```python
from build123d import *

# Parameters (mm, degrees)
EXTRUDE_1_DEPTH          = 15
CUT_EXTRUDE_1_DEPTH      = 15
CUT_EXTRUDE_1_DEPTH_BACK = 15
SKETCH_2_R               = 2.25
CUT_EXTRUDE_2_DEPTH      = 1.5
CUT_EXTRUDE_3_DEPTH      = 1.5
FILLET_1_R               = 0.5
FILLET_2_R               = 1


with BuildPart() as part:
    # Эскиз1 → Вытянуть1 (new body)
    with BuildSketch(Plane.XY):
        with BuildLine():
            Line((-25.229060352, 2.359412), (-25.229060352, 8.559412))
            ThreePointArc((-25.229060352, 8.559412), (-24.666370719, 9.730500928), (-23.400461317, 10.022977057))
            Line((-23.400461317, 10.022977057), (-5.12659913, 5.920136906))
            ThreePointArc((-5.12659913, 5.920136906), (-4.279542261, 5.877403833), (-3.466943303, 6.120332607))
            Line((-3.466943303, 6.120332607), (-1.866464924, 6.915175876))
            Line((-1.866464924, 6.915175876), (-1.510627877, 6.19867047))
            Line((-1.510627877, 6.19867047), (-3.111106257, 5.403827201))
            ThreePointArc((-3.111106257, 5.403827201), (-4.183736881, 5.083161219), (-5.301851949, 5.139568876))
            Line((-5.301851949, 5.139568876), (-23.575714136, 9.242409026))
            ThreePointArc((-23.575714136, 9.242409026), (-24.166471856, 9.105920166), (-24.429060352, 8.559412))
            Line((-24.429060352, 8.559412), (-24.429060352, 2.359412))
            ThreePointArc((-24.429060352, 2.359412), (-25.102714755, 0.733066403), (-26.729060352, 0.059412))
            Line((-26.729060352, 0.059412), (-33.229060352, 0.059412))
            Line((-33.229060352, 0.059412), (-33.229060352, 0.859412))
            Line((-33.229060352, 0.859412), (-26.729060352, 0.859412))
            ThreePointArc((-26.729060352, 0.859412), (-25.66840018, 1.298751828), (-25.229060352, 2.359412))
        make_face()
    extrude(amount=EXTRUDE_1_DEPTH)

    # Эскиз2 → Вырез-Вытянуть1 (cut, two sides: drawn at the far end of the back side and taken through both)
    with BuildSketch(Plane(origin=(0, 0.859412, 0), x_dir=(1, 0, 0), z_dir=(0, 1, 0)).offset(-CUT_EXTRUDE_1_DEPTH_BACK)):
        with Locations(Location((-29.629060352, -7.5, 0), (0, 0, 90))):
            Circle(SKETCH_2_R)
        Polygon((-13.229060352, -0.5), (-13.229060352, -2), (-0.791842207, -2), (-0.791842207, 0), (-26.729060352, 0), (-26.729060352, -0.5), align=None)
        Polygon((-26.729060352, -15), (-0.791842207, -15), (-0.791842207, -13), (-13.229060352, -13), (-13.229060352, -14.5), (-26.729060352, -14.5), align=None)
    extrude(amount=CUT_EXTRUDE_1_DEPTH + CUT_EXTRUDE_1_DEPTH_BACK, mode=Mode.SUBTRACT)

    # Эскиз3 → Вырез-Вытянуть2 (cut)
    with BuildSketch(Plane.XY.offset(14.5)):
        Polygon((-13.229060352, 7.739298224), (-13.229060352, 6.919382502), (-13.40431317, 6.958730194), align=None)
    extrude(amount=-CUT_EXTRUDE_2_DEPTH, mode=Mode.SUBTRACT)

    # Эскиз4 → Вырез-Вытянуть3 (cut)
    with BuildSketch(Plane(origin=(0, 0, 0.5), x_dir=(-1, 0, 0), z_dir=(0, 0, -1))):
        Polygon((13.229060352, 7.739298224), (13.229060352, 6.919382502), (13.40431317, 6.958730194), align=None)
    extrude(amount=-CUT_EXTRUDE_3_DEPTH, mode=Mode.SUBTRACT)

    # Скругление1
    # the kernel refuses this fillet: 0.5 mm, written as the material it adds along each edge
    with BuildSketch(Plane(origin=(-26.729060352, 2.109412, 14.5), x_dir=(0, 0, 1), z_dir=(0, -1, 0))) as fillet_1_piece_1_section:
        with BuildLine():
            CenterArc((FILLET_1_R, -FILLET_1_R), FILLET_1_R, 90, 90)
            Line((0, -FILLET_1_R), (0, 0))
            Line((0, 0), (FILLET_1_R, 0))
        make_face()
    fillet_1_piece_1 = extrude(amount=3.3, mode=Mode.PRIVATE)
    fillet_1_piece_1 = fillet_1_piece_1 - Plane(origin=(-26.729060352, 2.359412, 14.543282734), x_dir=(0, -1, 0), z_dir=(0, 0, -1)) * Cylinder(1.5, 9, mode=Mode.PRIVATE)
    fillet_1_piece_1 = fillet_1_piece_1 & Plane(origin=(-26.729060352, 2.359412, 14.543282734), x_dir=(1, 0, 0), z_dir=(0, 0, -1)) * Cylinder(2.3, 9, mode=Mode.PRIVATE)
    add(fillet_1_piece_1)
    with BuildSketch(Plane(origin=(-26.729060352, 2.109412, 0.5), x_dir=(0, 0, -1), z_dir=(0, -1, 0))) as fillet_1_piece_2_section:
        with BuildLine():
            CenterArc((FILLET_1_R, FILLET_1_R), FILLET_1_R, 180, 90)
            Line((0, FILLET_1_R), (0, 0))
            Line((0, 0), (FILLET_1_R, 0))
        make_face()
    fillet_1_piece_2 = extrude(amount=3.3, mode=Mode.PRIVATE)
    fillet_1_piece_2 = fillet_1_piece_2 - Plane(origin=(-26.729060352, 2.359412, 0.456717266), x_dir=(0, -1, 0), z_dir=(0, 0, -1)) * Cylinder(1.5, 9, mode=Mode.PRIVATE)
    fillet_1_piece_2 = fillet_1_piece_2 & Plane(origin=(-26.729060352, 2.359412, 0.456717266), x_dir=(1, 0, 0), z_dir=(0, 0, -1)) * Cylinder(2.3, 9, mode=Mode.PRIVATE)
    add(fillet_1_piece_2)

    # Скругление2
    fillet_2_edges = [part.edges().sort_by_distance(p)[0] for p in [
        (-1.6885464, 6.556923173, 13),
        (-13.316686761, 7.349014209, 13),
        (-13.316686761, 7.349014209, 2),
        (-1.6885464, 6.556923173, 2),
    ]]
    fillet(fillet_2_edges, radius=FILLET_2_R)


solid = part.part
```
Design review of the part built by this model. Coordinates are the model's own, in mm. A direction names the side the tool comes from. Give positions to 0.01 mm unless a question says otherwise; leave off trailing zeros. Loops run counter-clockwise (first coordinate to the right, second up) from the corner with the lowest first, then second, coordinate; pieces in that order, holes last. Notation, with made-up numbers: (17.5, 44.5) -> (45.5, 44.5) arc R5 ccw to (45.5, 52.5) -> close; hole circle Ø9 at (44, -30). An arc over 180 degrees is marked (long way). One line per item, written item: value.
Q1. For pin 1 Ø6 at (x, y) = (-19.5, 8) entering from -Z; pin 2 Ø4 at (x, y) = (-25.5, 5) entering from +Z; pin 3 Ø1.5 at (x, y) = (-9, 5.5) entering from -Z, all flat-tipped, find the tip position at first contact; note any pin that passes through.
Numbers:
pin 1: stops at z = 0.5
pin 2: stops at z = 14.5
pin 3: stops at z = 2
Q2. Machinability: for faces 1 (the flat face through (-32, 0.859, 7)), 2 (the flat face through (-14.39, 8, 7.4)), 3 (the flat face through (-7, 6, 13)), which of the approach directions +Z, -Z, +X, -X, +Y, -Y give a long, thin tool a straight path to every point of the face, cutting with its end or side? Answer none if there is none.
Numbers:
face 1: +Z, -Z, -X, +Y
face 2: +Z, -Z, +Y
face 3: +Z, +X, +Y, -Y
Q3. We need section B-B on x = -30.5. Give the boundary of the cut face in (y, z), and give its area (3 significant figures).
Numbers:
outline: (0.06, 0) -> (0.86, 0) -> (0.86, 5.43) -> (0.06, 5.43) -> close; (0.06, 9.57) -> (0.86, 9.57) -> (0.86, 15) -> (0.06, 15) -> close
area: 8.68 mm^2
Q4. We need section A-A on z = 7.5. Give the boundary of the cut face in (x, y).
Numbers:
outline: (-33.23, 0.06) -> (-31.88, 0.06) -> (-31.88, 0.86) -> (-33.23, 0.86) -> close; (-27.38, 0.06) -> (-26.73, 0.06) arc R2.3 ccw to (-24.43, 2.36) -> (-24.43, 8.56) arc R0.7 cw to (-23.58, 9.24) -> (-5.3, 5.14) arc R3.3 ccw to (-3.11, 5.4) -> (-1.51, 6.2) -> (-1.87, 6.92) -> (-3.47, 6.12) arc R2.5 cw to (-5.13, 5.92) -> (-23.4, 10.02) arc R1.5 ccw to (-25.23, 8.56) -> (-25.23, 2.36) arc R1.5 cw to (-26.73, 0.86) -> (-27.38, 0.86) -> close
Q5. We need section C-C on z = 10.75. Give the boundary of the cut face in (x, y).
Numbers:
outline: (-33.23, 0.06) -> (-26.73, 0.06) arc R2.3 ccw to (-24.43, 2.36) -> (-24.43, 8.56) arc R0.7 cw to (-23.58, 9.24) -> (-5.3, 5.14) arc R3.3 ccw to (-3.11, 5.4) -> (-1.51, 6.2) -> (-1.87, 6.92) -> (-3.47, 6.12) arc R2.5 cw to (-5.13, 5.92) -> (-23.4, 10.02) arc R1.5 ccw to (-25.23, 8.56) -> (-25.23, 2.36) arc R1.5 cw to (-26.73, 0.86) -> (-33.23, 0.86) -> close
Q6. For L1, parallel to X at y = 0.3, z = 7.5; L2, parallel to X at y = 0.7, z = 7.5; L3, parallel to Z at x = -25, y = 6, list the stretches that pass through material, from the lowest coordinate up.
Numbers:
L1: x = -33.23 to -31.88, -27.38 to -25.7
L2: x = -33.23 to -31.88, -27.38 to -25.14
L3: z = 0.5 to 14.5
Q7. Draft analysis for pull direction X (two halves, no side actions). For faces 4 (the flat face through (-21, 9, 0.5)), 5 (the cylindrical face through (-24.16, 9.11, 7.4)), 6 (the cylindrical face through (-1.955, 6.418, 12.715)), 7 (the flat face through (-2.7, 6.5, 7.4)), state which applies: pulls with the +X half, pulls with the -X half, needs draft (parallel to the pull), parting line crosses it, or undercut.
Numbers:
face 4: needs draft
face 5: undercut
face 6: pulls with the +X half
face 7: undercut
Q8. We need section D-D on x = -17. Give the boundary of the cut face in (y, z).
Numbers:
outline: (7.77, 0.5) -> (8.59, 0.5) -> (8.59, 14.5) -> (7.77, 14.5) -> close
